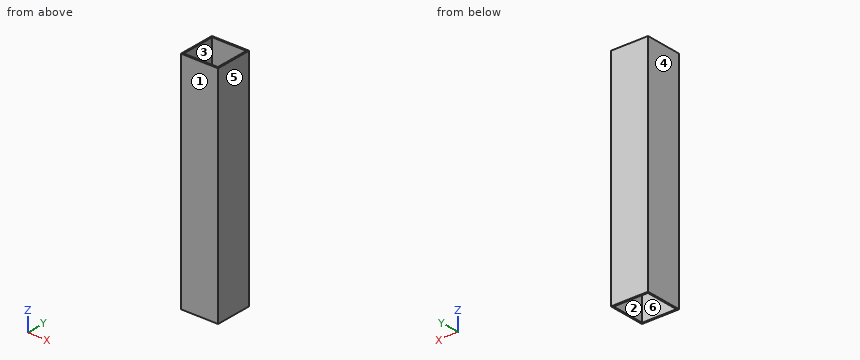
Autodesk Inventor part; units mm, degrees
ref_plane "YZ Plane" through (0, 0, 0) normal (1, 0, 0) x (0, 1, 0)
ref_plane "XZ Plane" through (0, 0, 0) normal (0, 1, 0) x (-1, 0, 0)
ref_plane "XY Plane" through (0, 0, 0) normal (0, 0, 1) x (1, 0, 0)
sketch "Boceto1" plane through (0, 0, 0) normal (0, 0, 1) x (1, 0, 0)
  line L0 (-37.5, 37.5) -> (37.5, 37.5)
  line L1 (37.5, 37.5) -> (37.5, -37.5)
  line L2 (37.5, -37.5) -> (-37.5, -37.5)
  line L3 (-37.5, -37.5) -> (-37.5, 37.5)
  line L4 (34.5, 34.5) -> (-34.5, 34.5)
  line L5 (-34.5, 34.5) -> (-34.5, -34.5)
  line L6 (-34.5, -34.5) -> (34.5, -34.5)
  line L7 (34.5, -34.5) -> (34.5, 34.5)
  point P0 (0, 0)
  dimension "d0" = 75
  dimension "d1" = 75
  dimension "d2" = 3
  dimension "d3" = 37.5
  dimension "d4" = 37.5
extrude "Extrusión1" add sketch "Boceto1" along normal mid plane 450
equation "\"d0\" = width"
equation "\"d1\" = height"
equation "\"d2\" = t"
equation "\"d5\" = length"
equation "\"width\" = 75"
equation "\"height\" = 75"
equation "\"t\" = 3"
equation "\"length\" = 450"
properties part number "45 STEEL PROFILE" material "Acero"
For this review, take the finished solid that the model builds, in its own axes (mm). Face numbers are marked on the shaded views. A direction names the side the tool comes from. Coordinates: 2 decimals unless noted, no trailing zeros. Loops run counter-clockwise (first coordinate to the right, second up) from the corner with the lowest first, then second, coordinate; pieces in that order, holes last.
1. Add section A-A, the plane x = -12. Give the boundary of the cut face in (y, z), then the cut area to 3 significant figures.
2. Add section C-C, the plane z = 76.5. Give the boundary of the cut face in (x, y), then the cut area to 3 significant figures.
3. Mouldability with a two-part tool opening along Y and no side actions: class the marked faces 1, 2, 3 and 4 as +Y half, -Y half, draft (parallel to the pull), parting line (faces both ways), or undercut.
4. For line 1 (Y direction, x = -15, z = 114), list the stretches that pass through material, from the lowest coordinate up.
5. For the marked faces 5 and 6, list the 3-axis set-ups (+Z, -Z, +X, -X, +Y, -Y) from which the entire face can be reached by the end or side of a thin tool; tool diameter is ignored.
Result:
1. outline: (-37.5, -225) - (-34.5, -225) - (-34.5, 225) - (-37.5, 225) - close; (34.5, -225) - (37.5, -225) - (37.5, 225) - (34.5, 225) - close
1. area: 2,700 mm2
2. outline: (-37.5, -37.5) - (37.5, -37.5) - (37.5, 37.5) - (-37.5, 37.5) - close; hole (-34.5, -34.5) - (34.5, -34.5) - (34.5, 34.5) - (-34.5, 34.5) - close
2. area: 864 mm2
3. face 1: -Y half
3. face 2: undercut
3. face 3: undercut
3. face 4: draft
4. line 1: y = -37.5 to -34.5, 34.5 to 37.5
5. face 5: +Z, -Z, +X, +Y, -Y
5. face 6: +Z, -Z
